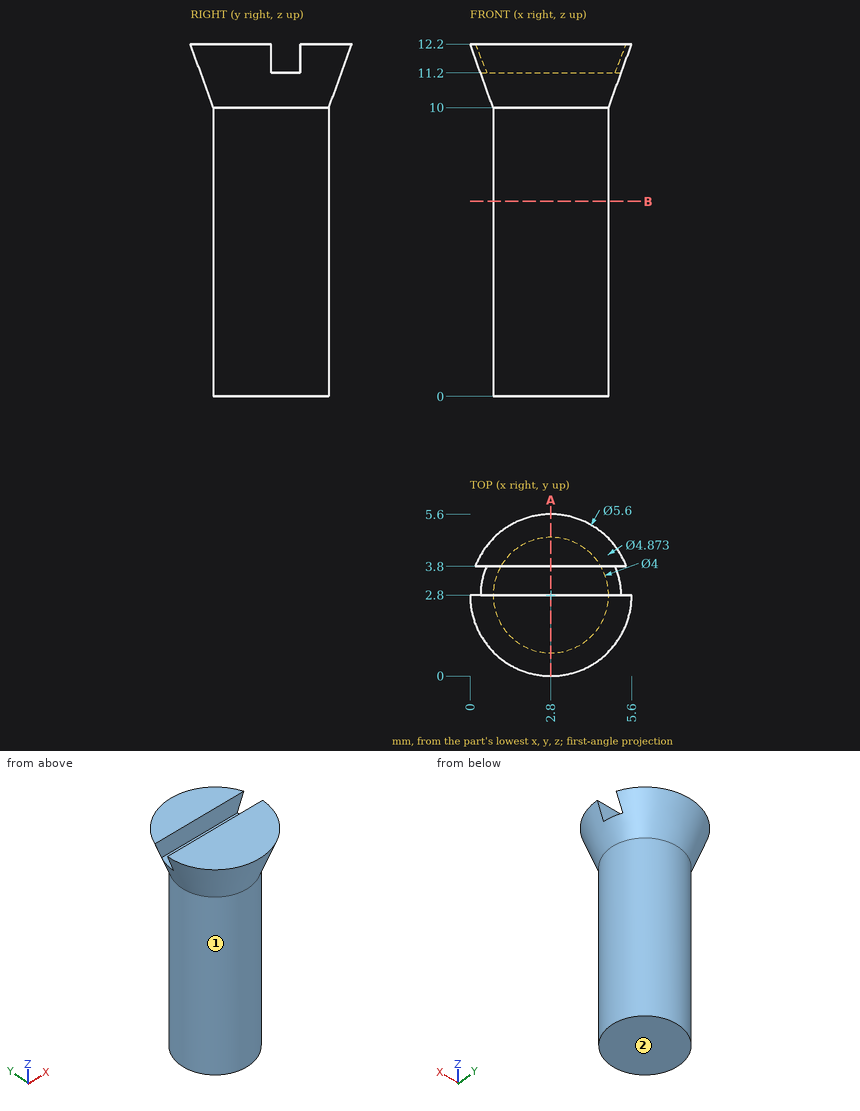
Geometry check sheet. Reference: drawing and pictorial views, mm from the part's lowest x, y, z. A direction names the side the tool comes from. Give positions to 0.01 mm unless a question says otherwise; leave off trailing zeros. Order: outer loops, then holes, each group sorted by start corner. A loop starts at its lowest first (then second) coordinate and runs counter-clockwise, first axis right, second up. Notation, with made-up numbers: M -20.5,-3.5 L 4.5,-3.5 A31 ccw 4.5,31.5 Z; hole C -14.75,7 d4. An arc over 180 degrees is marked long. Answer in a Markdown table with one row per item. Add a question column.
Q1. Sectioned sample at A-A, the plane x = 2.8. Record the boundary of the cut face in (y, z).
Q2. Access from +Z, -Z, +X, -X, +Y, -Y to the whole of each face (thin tool, end or side, straight path). Record for the marked faces 1 and 2.
Q3. Sectioned sample at B-B, the plane z = 6.75. Record the boundary of the cut face in (x, y).
Q4. Gauge pin test, flat end, axial feed: pin 1 Ø1.5 at (y, z) = (4, 7.5) entering from -X. Record the tip position at first contact, or that the pin passes through.
Q5. Thickness scan on L1, parallel to X at y = 2.85, z = 2.75; L2, parallel to Z at x = 4.4, y = 2.9; L3, parallel to X at y = 3.95, z = 1.5 (1 decimal). Record the ranges inside material, lowest first.
Verdict:
| question | item | result |
|---|---|---|
| 1 | outline | M 0,12.2 L 0.8,10 L 0.8,0 L 4.8,0 L 4.8,10 L 5.6,12.2 L 3.8,12.2 L 3.8,11.2 L 2.8,11.2 L 2.8,12.2 Z |
| 2 | face 1 | -Z |
| 2 | face 2 | -Z, +X, -X, +Y, -Y |
| 3 | outline | C 2.8,2.8 d4 |
| 4 | pin 1 | x = 0.85 |
| 5 | L1 | 0.8 to 4.8 |
| 5 | L2 | 0 to 11.2 |
| 5 | L3 | 1.2 to 4.4 |
